Input: dimensioned drawing with shaded views. Units: mm. Origin: part minimum x, y, z. Round coordinates to 2 decimals unless told otherwise and drop trailing zeros. Write each loop counter-clockwise with the first axis right and the second up, starting at its lowest first coordinate (ties: lowest second). Pieces come first, ordered by that corner, then holes. Notation, with made-up numbers: (62.5, -25) -> (88.5, -25) arc R11 cw to (88.5, -21) -> close; hole circle Ø1 at (48, -30.5). An arc over 180 degrees is marked (long way). Use one line per item in the form item = value. Start each with the question number.
1. Cut plane B-B, the plane x = 7.5. Return the cut outline in (y, z).
2. Cut plane D-D, the plane y = 1. Return the cut outline in (x, z).
3. Cut plane C-C, the plane z = 0.8. Return the cut outline in (x, y).
4. Cut plane A-A, the plane y = 5. Return the cut outline in (x, z).
5. Line query: L1, parallel to Y at x = 37.5, z = 1.75; L2, parallel to X at y = 4.5, z = 0.75; L3, parallel to X at y = 5.75, z = 2.45. Output: solid intervals per line, ascending.
6. Pin query (flat end, axial travel): pin 1 Ø2 at (x, y) = (7.5, 5) entering from +Z. Return the tip coordinate at first contact, or that it passes through.
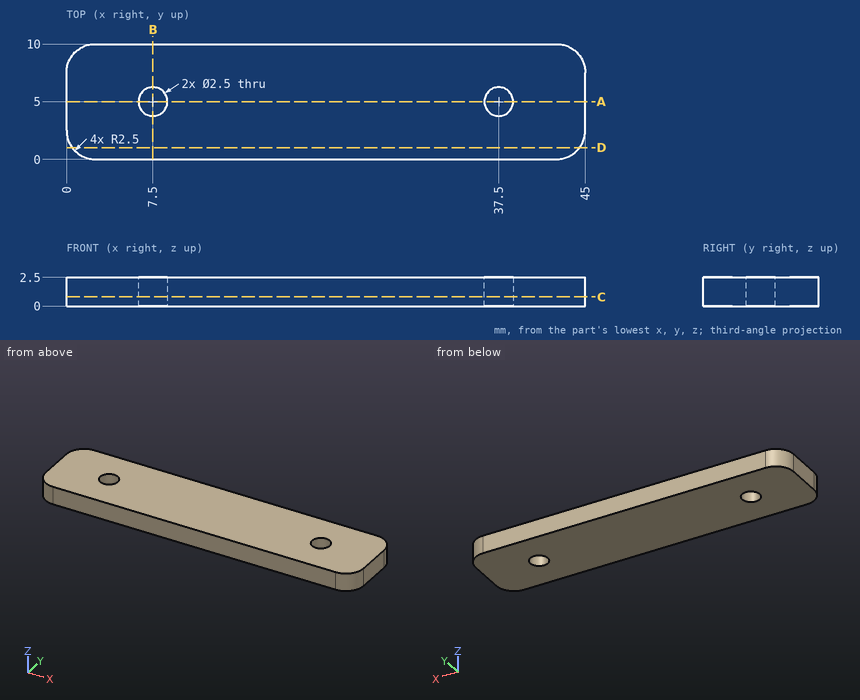
Outcome:
q1.outline = (0, 0) -> (3.75, 0) -> (3.75, 2.5) -> (0, 2.5) -> close; (6.25, 0) -> (10, 0) -> (10, 2.5) -> (6.25, 2.5) -> close
q2.outline = (0.5, 0) -> (44.5, 0) -> (44.5, 2.5) -> (0.5, 2.5) -> close
q3.outline = (0, 2.5) arc R2.5 ccw to (2.5, 0) -> (42.5, 0) arc R2.5 ccw to (45, 2.5) -> (45, 7.5) arc R2.5 ccw to (42.5, 10) -> (2.5, 10) arc R2.5 ccw to (0, 7.5) -> close; hole circle Ø2.5 at (7.5, 5); hole circle Ø2.5 at (37.5, 5)
q4.outline = (0, 0) -> (6.25, 0) -> (6.25, 2.5) -> (0, 2.5) -> close; (8.75, 0) -> (36.25, 0) -> (36.25, 2.5) -> (8.75, 2.5) -> close; (38.75, 0) -> (45, 0) -> (45, 2.5) -> (38.75, 2.5) -> close
q5.L1 = 0 to 3.75, 6.25 to 10
q5.L2 = 0 to 6.35, 8.65 to 36.35, 38.65 to 45
q5.L3 = 0 to 6.5, 8.5 to 36.5, 38.5 to 45
q6.pin_1 = through
